Can you work these out from the model? Positions are in its coordinate system, mm. Face numbers are marked on the shaded views. Round coordinates to 2 decimals unless told otherwise and drop trailing zeros. Order: outer loops, then holes, each group sorted by start corner. A loop starts at its lowest first (then second) coordinate and runs counter-clockwise, first axis right, second up. Notation, with made-up numbers: (46.25, -30.75) -> (87.25, -30.75) arc R24 ccw to (87.25, 2.25) -> close; hole circle Ø8 at (-2.75, 64). An arc over 180 degrees is marked (long way). Use a Markdown table: item, result. Add a question column.
Q1. If we section it at B-B on x = 5: List the corners of the cut face in (y, z) for me.
Q2. If we section it at D-D on z = 11.75: List the corners of the cut face in (x, y) for me.
Q3. We'd pull the mould along Y, two halves only. Please class the marked faces 1, 2 and 3: +Y half, -Y half, draft (parallel to the pull), parting line (faces both ways), or undercut.
Q4. I'm going to push flat-ended pins straight in: pin 1 Ø1.5 at (x, z) = (-29.5, 16.5) entering from +Y; pin 2 Ø5 at (y, z) = (32, 12.5) entering from +X; pin 3 Ø11 at (x, y) = (0, 0) entering from -Z; pin 4 Ø1.5 at (y, z) = (-0.5, 17) entering from -X. Where does each tip first touch, or does it pass through?
Q5. If we section it at A-A on y = -20: List the corners of the cut face in (x, z) for me, plus the area to 3 significant figures.
Q6. I need wall thicknesses on line 1 along Y through (x, z) = (0, 12.5); line 2 along Z through (x, y) = (12.5, -22.5); line 3 along Z through (x, y) = (-38.8, 0). Which ranges of each line are inside material? Lowest first, please. Write a range as [from, to].
Q7. If we section it at C-C on y = 0: List the corners of the cut face in (x, z) for me.
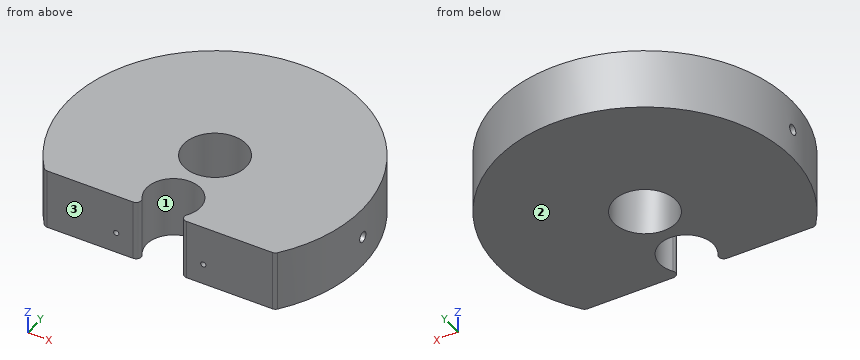
```python
from build123d import *

# Parameters (mm, degrees)
SKETCH007_R     = 9
PAD005_DEPTH    = 17.5
FILLET_R        = 1.5
SKETCH022_R     = 1.5
POCKET010_DEPTH = 5
SKETCH023_R     = 0.75
POCKET011_DEPTH = 10
SKETCH026_R     = 1.5
POCKET014_DEPTH = 5


with BuildPart() as part:
    # Sketch007 → Pad005 (new body)
    with BuildSketch(Plane.XY):
        with BuildLine():
            Line((-33.051802, -26.637959), (-4, -26.637959))
            ThreePointArc((4, -26.637959), (0, -12.25), (-4, -26.637959))
            Line((33.051802, -26.637959), (4, -26.637959))
            ThreePointArc((33.051802, -26.637959), (0, 42.45), (-33.051802, -26.637959))
        make_face()
        Circle(SKETCH007_R, mode=Mode.SUBTRACT)
    extrude(amount=PAD005_DEPTH)

    # Fillet
    fillet_edges = [part.edges().sort_by_distance(p)[0] for p in [
        (-4, -26.637959, 8.75),
        (4, -26.637959, 8.75),
        (-33.051802, -26.637959, 8.75),
        (33.051802, -26.637959, 8.75),
    ]]
    fillet(fillet_edges, radius=FILLET_R)

    # Sketch022 (on DatumPlane) → Pocket010 (cut)
    with BuildSketch(Plane.YZ.offset(42.45)):
        with Locations((0, 8.75)):
            Circle(SKETCH022_R)
    extrude(amount=-POCKET010_DEPTH, mode=Mode.SUBTRACT)

    # Sketch023 (on DatumPlane) → Pocket011 (cut)
    with BuildSketch(Plane.XZ.offset(26.7)):
        with Locations((12.5, 6)):
            Circle(SKETCH023_R)
        with Locations((-12.5, 6)):
            Circle(SKETCH023_R)
    extrude(amount=-POCKET011_DEPTH, mode=Mode.SUBTRACT)

    # Sketch026 (on DatumPlane) → Pocket014 (cut)
    with BuildSketch(Plane.YZ.offset(-42.45)):
        with Locations((0, 8.75)):
            Circle(SKETCH026_R)
    extrude(amount=POCKET014_DEPTH, mode=Mode.SUBTRACT)


with BuildPart() as part_1:
    # Body005 placement: moved
    add(part.part.moved(Location((0, 0, 8))))


solid = part_1.part
```
Answer below:
| question | item | result |
|---|---|---|
| 1 | outline | (-14.08, 8) -> (-7.48, 8) -> (-7.48, 25.5) -> (-14.08, 25.5) -> close; (7.48, 8) -> (42.15, 8) -> (42.15, 25.5) -> (7.48, 25.5) -> close |
| 2 | outline | (-33.51, -26.06) arc R1.5 ccw to (-32.33, -26.64) -> (-7.69, -26.64) arc R1.5 ccw to (-6.44, -24.3) arc R7.75 cw (long way) to (6.44, -24.3) arc R1.5 ccw to (7.69, -26.64) -> (32.33, -26.64) arc R1.5 ccw to (33.51, -26.06) arc R42.45 ccw (long way) to start; hole circle Ø18 at (0, 0) |
| 3 | face 1 | undercut |
| 3 | face 2 | draft |
| 3 | face 3 | -Y half |
| 4 | pin 1 | y = 31.23 |
| 4 | pin 2 | x = 30.52 |
| 4 | pin 3 | through |
| 4 | pin 4 | x = -37.45 |
| 5 | outline | (-37.44, 8) -> (-7.75, 8) -> (-7.75, 25.5) -> (-37.44, 25.5) -> close; (7.75, 8) -> (37.44, 8) -> (37.44, 25.5) -> (7.75, 25.5) -> close; hole circle Ø1.5 at (-12.5, 14); hole circle Ø1.5 at (12.5, 14) |
| 5 | area | 1,040 mm² |
| 6 | line 1 | [-12.25, -9], [9, 42.45] |
| 6 | line 2 | [8, 13.25], [14.75, 25.5] |
| 6 | line 3 | [8, 15.25], [18.25, 25.5] |
| 7 | outline | (-42.45, 8) -> (-9, 8) -> (-9, 25.5) -> (-42.45, 25.5) -> (-42.45, 18.25) -> (-37.45, 18.25) -> (-37.45, 15.25) -> (-42.45, 15.25) -> close; (9, 8) -> (42.45, 8) -> (42.45, 15.25) -> (37.45, 15.25) -> (37.45, 18.25) -> (42.45, 18.25) -> (42.45, 25.5) -> (9, 25.5) -> close |
